```python
from build123d import *

# Parameters (mm, degrees)
SKETCH_W        = 16
SKETCH_H        = 20
PAD_DEPTH       = 2
POCKET_DEPTH    = 2
SKETCH002_W     = 8
SKETCH002_H     = 2
SKETCH002_W_2   = 2
SKETCH002_H_2   = 8
SKETCH002_W_3   = 4
SKETCH002_H_3   = 6
PAD001_DEPTH    = 2
POCKET001_DEPTH = 2
POCKET002_DEPTH = 2
FILLET_R        = 3
SKETCH005_R     = 1
POCKET003_DEPTH = 2
SKETCH006_W     = 2
SKETCH006_H     = 10
PAD002_DEPTH    = 2
POCKET004_DEPTH = 2


with BuildPart() as part:
    # Sketch → Pad (new body)
    with BuildSketch(Plane.XY):
        with Locations((8, 10)):
            Rectangle(SKETCH_W, SKETCH_H)
    extrude(amount=PAD_DEPTH)

    # Sketch001 (on Face6 of Pad) → Pocket (cut)
    with BuildSketch(Plane.XY.offset(2)):
        Polygon((8, 0), (16, 0), (16, 8), align=None)
    extrude(amount=-POCKET_DEPTH, mode=Mode.SUBTRACT)

    # Sketch002 (on Face4 of Pocket) → Pad001 (join)
    with BuildSketch(Plane.XY.offset(2)):
        with Locations((4, 1)):
            Rectangle(SKETCH002_W, SKETCH002_H)
        with Locations((15, 16)):
            Rectangle(SKETCH002_W_2, SKETCH002_H_2)
        with Locations((12, 19)):
            Rectangle(SKETCH002_W_3, SKETCH002_H)
        with Locations((1, 5)):
            Rectangle(SKETCH002_W_2, SKETCH002_H_3)
    extrude(amount=PAD001_DEPTH)

    # Sketch003 (on Face17 of Pad001) → Pocket001 (cut)
    with BuildSketch(Plane.XZ.offset(-18)):
        Polygon((10, 2), (14, 4), (10, 4), align=None)
    extrude(amount=-POCKET001_DEPTH, mode=Mode.SUBTRACT)

    # Sketch004 (on Face21 of Pocket001) → Pocket002 (cut)
    with BuildSketch(Plane.YZ.offset(2)):
        Polygon((2, 4), (8, 2), (8, 4), align=None)
    extrude(amount=-POCKET002_DEPTH, mode=Mode.SUBTRACT)

    # Fillet
    fillet_edges = [part.edges().sort_by_distance(p)[0] for p in [
        (0, 20, 1),
    ]]
    fillet(fillet_edges, radius=FILLET_R)

    # Sketch005 (on Face8 of Fillet) → Pocket003 (cut)
    with BuildSketch(Plane.XY.offset(2)):
        with Locations((3, 17)):
            Circle(SKETCH005_R)
    extrude(amount=-POCKET003_DEPTH, mode=Mode.SUBTRACT)

    # Sketch006 (on Face9 of Pocket003) → Pad002 (join)
    with BuildSketch(Plane.XY.offset(2)):
        with Locations((8, 11)):
            Rectangle(SKETCH006_W, SKETCH006_H)
    extrude(amount=PAD002_DEPTH)

    # Sketch007 (on Face25 of Pad002) → Pocket004 (cut)
    with BuildSketch(Plane.YZ.offset(9)):
        Polygon((9, 4), (13, 4), (11, 3), align=None)
    extrude(amount=-POCKET004_DEPTH, mode=Mode.SUBTRACT)


solid = part.part
```
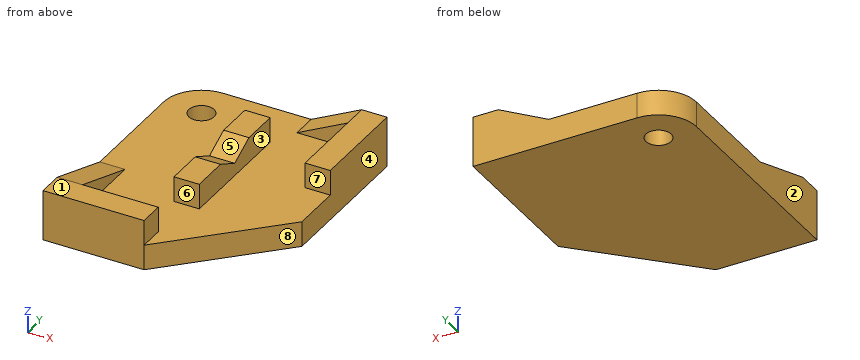
Source: CAD feature listing. Evaluate the final solid. Frame: model axes, mm. Face numbers are marked on the shaded views. A direction names the side the tool comes from. Round coordinates to 2 decimals unless told otherwise and drop trailing zeros. Loops run counter-clockwise (first coordinate to the right, second up) from the corner with the lowest first, then second, coordinate; pieces in that order, holes last. Notation, with made-up numbers: (4.5, 71.25) - (12.5, 71.25) arc R32 ccw to (12.5, 97.25) - close; hole circle Ø11 at (62, 34.5). An arc over 180 degrees is marked (long way). Use CSV: the item, a comma, the result in double quotes.
Q1. Section query B-B, the plane x = 4.75. Output: boundary loops of the cut face in (y, z).
Reported:
outline,"(0, 0) - (20, 0) - (20, 2) - (2, 2) - (2, 4) - (0, 4) - close"
Q2. Section query C-C, the plane y = 3. Output: boundary loops of the cut face in (x, z), then the cut area to 3 significant figures.
Reported:
outline,"(0, 0) - (11, 0) - (11, 2) - (2, 2) - (2, 3.67) - (0, 3.67) - close"
area,"25.3 mm^2"
Q3. Pin query (flat end, axial travel): pin 1 Ø1 at (y, z) = (5, 3) entering from +X; pin 2 Ø1.6 at (y, z) = (11.5, 3) entering from -X; pin 3 Ø0.6 at (y, z) = (11.5, 3) entering from +X; pin 4 Ø1.2 at (x, y) = (3, 17) entering from -Z. Return the tip coordinate at first contact, or that it passes through.
Reported:
pin 1,"x = 2"
pin 2,"x = 7"
pin 3,"x = 9"
pin 4,"through"
Q4. Section query D-D, the plane y = 9.75. Output: boundary loops of the cut face in (x, z) (3 decimals).
Reported:
outline,"(0, 0) - (16, 0) - (16, 2) - (9, 2) - (9, 3.625) - (7, 3.625) - (7, 2) - (0, 2) - close"
Q5. Mould query, pull axis X, two halves, no side actions, for the marked faces 1, 2, 3 and 4. Classes: pulls with the +X half, pulls with the -X half, needs draft (parallel to the pull), parting line crosses it, or undercut.
Reported:
face 1,"needs draft"
face 2,"pulls with the -X half"
face 3,"undercut"
face 4,"pulls with the +X half"
Q6. Ray query, line 1 along Y through (x, z) = (3, 1); line 2 along X through (y, z) = (17, 2.45); line 3 along Z through (x, y) = (1, 5). Return the intervals inside material, ascending.
Reported:
line 1,"0 to 16, 18 to 20"
line 2,"14 to 16"
line 3,"0 to 3"
Q7. Section query A-A, the plane z = 1.4. Output: boundary loops of the cut face in (x, y).
Reported:
outline,"(0, 0) - (8, 0) - (16, 8) - (16, 20) - (3, 20) arc R3 ccw to (0, 17) - close; hole circle Ø2 at (3, 17)"
Q8. Reachability of the marked faces 5, 6, 7 and 8 from +Z, -Z, +X, -X, +Y, -Y: full face, straight path, thin tool, end or side. Return the list, or none.
Reported:
face 5,"+Z, -X"
face 6,"+Z, +X"
face 7,"+Z, +X, -Y"
face 8,"+Z, -Z, +X, -Y"
